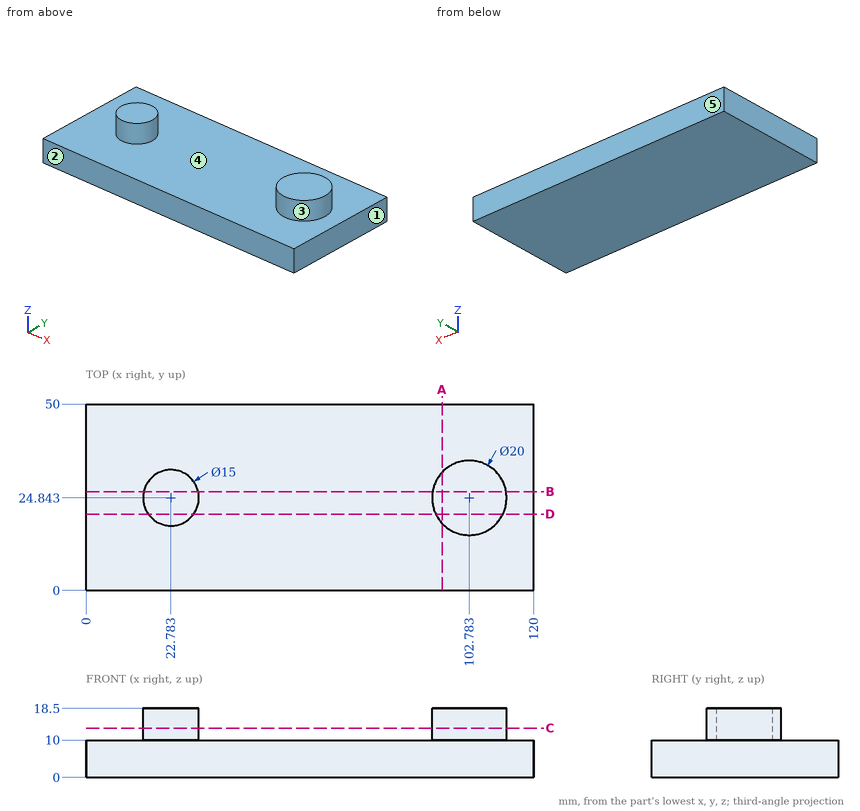
Here's the drawing with two shaded views (mm, measured from the low corner). I have some questions. A direction names the side the tool comes from. Coordinates: 2 decimals unless noted, no trailing zeros. Loops run counter-clockwise (first coordinate to the right, second up) from the corner with the lowest first, then second, coordinate; pieces in that order, holes last. Notation, with made-up numbers: M -1.5,17.5 L 18.5,17.5 A15 ccw 18.5,24.5 Z; hole C -13,-35.75 d8. An arc over 180 degrees is marked long. Return JSON: item names as keys, results as strings. Group by question number.
Item 1: I'm going to push flat-ended pins straight in: pin 1 Ø8 at (x, y) = (18.5, 8) entering from +Z; pin 2 Ø1 at (y, z) = (34, 12) entering from -X. Where does each tip first touch, or does it pass through?
Item 2: Imagine slicing it at A-A (x = 95.5). Please give me the cut outline in (y, z).
Item 3: Thinking about a two-plate mould opening in X: for the marked faces 1, 2 and 3, which applies, released by +X, released by -X, zero draft, split by the parting line, or undercut?
Item 4: On a 3-axis mill with a long thin cutter (end or side, diameter ignored), from which of +Z, -Z, +X, -X, +Y, -Y can I reach the whole of each face in a straight line? I mean the marked faces 4 and 5. Say none if no direction works.
Item 5: If I drill on L1, parallel to Z at x = 83, y = 27; L2, parallel to Y at x = 108, z = 13.75 (1 decimal); L3, parallel to X at y = 29.5, z = 13 (1 decimal), over which ranges is the centre line in solid material (lowest first)? Write a range as from..to.
Item 6: Imagine slicing it at C-C (z = 13.25). Please give me the cut outline in (x, y).
Item 7: Imagine slicing it at B-B (y = 26.5). Please give me the cut outline in (x, z) (1 decimal), and give its area (3 significant figures).
Item 8: Imagine slicing it at D-D (y = 20.5). Please give me the cut outline in (x, z) (1 decimal).
Verdict:
{
 "1": {"pin 1": "stops at z = 10", "pin 2": "stops at x = 97.78"},
 "2": {"outline": "M 0,0 L 50,0 L 50,10 L 31.7,10 L 31.7,18.5 L 17.99,18.5 L 17.99,10 L 0,10 Z"},
 "3": {"face 1": "released by +X", "face 2": "zero draft", "face 3": "undercut"},
 "4": {"face 4": "+Z", "face 5": "+Z, -Z, +X, -X, +Y"},
 "5": {"L1": "z = 0..10", "L2": "y = 16.3..33.4", "L3": "x = 16.9..28.7, 93.9..111.6"},
 "6": {"outline": "C 22.78,24.84 d15; C 102.78,24.84 d20"},
 "7": {"outline": "M 0,0 L 120,0 L 120,10 L 112.6,10 L 112.6,18.5 L 92.9,18.5 L 92.9,10 L 30.1,10 L 30.1,18.5 L 15.5,18.5 L 15.5,10 L 0,10 Z", "area": "1,490 mm^2"},
 "8": {"outline": "M 0,0 L 120,0 L 120,10 L 111.8,10 L 111.8,18.5 L 93.8,18.5 L 93.8,10 L 28.9,10 L 28.9,18.5 L 16.7,18.5 L 16.7,10 L 0,10 Z"}
}
